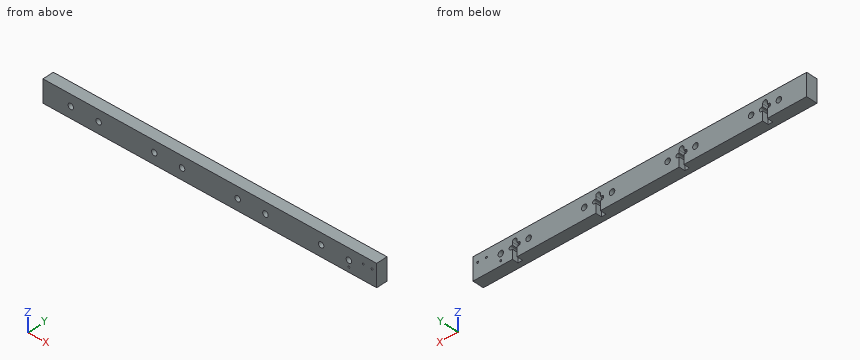
from build123d import *

# Parameters (mm, degrees)
SKETCH1_W                = 360
SKETCH1_H                = 24
BOSS_EXTRUDE1_DEPTH      = 12
CUT_EXTRUDE1_REACH       = 182.798
SKETCH2_R                = 3
CUT_EXTRUDE2_DEPTH       = 8
CUT_EXTRUDE3_DEPTH       = 6.5
LPATTERN1_COUNT          = 4
LPATTERN1_PITCH          = 90
F_2_0_2_DIAMETER_HOLE1_D = 2


with BuildPart() as part:
    # Sketch1 → Boss-Extrude1 (new body)
    with BuildSketch(Plane(origin=(0, 0, 0), x_dir=(1, 0, 0), z_dir=(0, 1, 0))):
        Rectangle(SKETCH1_W, SKETCH1_H)
    extrude(amount=BOSS_EXTRUDE1_DEPTH)

    # Sketch2 → Cut-Extrude1 (cut, up to next)
    with BuildSketch(Plane(origin=(0, 12, 0), x_dir=(1, 0, 0), z_dir=(0, 1, 0)), mode=Mode.PRIVATE) as cut_extrude1_sk1:
        with Locations(Location((-150, 0, 0), (0, 0, 270))):
            Circle(SKETCH2_R)
    cut_extrude1_tool1 = extrude(cut_extrude1_sk1.sketch, amount=-CUT_EXTRUDE1_REACH, mode=Mode.PRIVATE) & part.part
    # Sketch2 → Cut-Extrude1 (cut, up to next)
    with BuildSketch(Plane(origin=(0, 12, 0), x_dir=(1, 0, 0), z_dir=(0, 1, 0)), mode=Mode.PRIVATE) as cut_extrude1_sk2:
        with Locations(Location((-120, 0, 0), (0, 0, 270))):
            Circle(SKETCH2_R)
    cut_extrude1_tool2 = extrude(cut_extrude1_sk2.sketch, amount=-CUT_EXTRUDE1_REACH, mode=Mode.PRIVATE) & part.part
    cut_extrude1_1 = cut_extrude1_tool1.solids().sort_by_distance((-150, 12, 0))[0]
    add(cut_extrude1_1, mode=Mode.SUBTRACT)
    cut_extrude1_2 = cut_extrude1_tool2.solids().sort_by_distance((-120, 12, 0))[0]
    add(cut_extrude1_2, mode=Mode.SUBTRACT)
    cut_extrude1 = cut_extrude1_1 + cut_extrude1_2  # Cut-Extrude1 as one shape, for the pattern or mirror that repeats it

    # Sketch11 → Cut-Extrude2 (cut)
    with BuildSketch(Plane(origin=(-63.484819349, 12, 93.481372316), x_dir=(-1, 0, 0), z_dir=(0, 1, 0))):
        with BuildLine():
            Line((67.515180651, -91.481372316), (75.515180651, -91.481372316))
            ThreePointArc((75.515180651, -91.481372316), (77.515180651, -93.481372316), (75.515180651, -95.481372316))
            Line((75.515180651, -95.481372316), (67.515180651, -95.481372316))
            ThreePointArc((67.515180651, -95.481372316), (65.515180651, -93.481372316), (67.515180651, -91.481372316))
        make_face()
    cut_extrude2 = extrude(amount=-CUT_EXTRUDE2_DEPTH, mode=Mode.SUBTRACT)

    # Sketch13 → Cut-Extrude3 (cut)
    with BuildSketch(Plane(origin=(-63.484819349, 12, 93.481372316), x_dir=(-1, 0, 0), z_dir=(0, 1, 0))):
        with BuildLine():
            Line((74.015180651, -88.481372316), (74.015180651, -142.11123171))
            ThreePointArc((74.015180651, -142.11123171), (71.515180651, -144.61123171), (69.015180651, -142.11123171))
            Line((69.015180651, -142.11123171), (69.015180651, -88.481372316))
            ThreePointArc((69.015180651, -88.481372316), (71.515180651, -85.981372316), (74.015180651, -88.481372316))
        make_face()
    cut_extrude3 = extrude(amount=-CUT_EXTRUDE3_DEPTH, mode=Mode.SUBTRACT)

    # LPattern1: Cut-Extrude1, Cut-Extrude2, Cut-Extrude3 ×4
    with Locations(*[(i * LPATTERN1_PITCH, 0, 0) for i in range(1, LPATTERN1_COUNT)]):
        add(cut_extrude1, mode=Mode.SUBTRACT)
        add(cut_extrude2, mode=Mode.SUBTRACT)
        add(cut_extrude3, mode=Mode.SUBTRACT)

    # Ø2.0 (2) Diameter Hole1 (through all)
    with Locations(Plane.XZ):
        with Locations((165.5, 4), (175, 4), (150, -7)):
            Hole(F_2_0_2_DIAMETER_HOLE1_D / 2)


solid = part.part
Check sheet for the modelled part. Datum: model origin and axes. Units: mm. Round coordinates to 2 decimals unless told otherwise and drop trailing zeros. Order: outer loops, then holes, each group sorted by start corner. A loop starts at its lowest first (then second) coordinate and runs counter-clockwise, first axis right, second up.
(1) Cross-section at A-A, the plane x = 120. Enter the section's corners in (y, z).
(2) Cross-section at B-B, the plane y = 7.5. State how many separate pieces and enclosed holes the cut face has, and give its area (3 significant figures).
(3) Scan lines: probe 1 along Z at (x, y) = (30, 5.5); probe 2 along X at (y, z) = (10.5, -5.5); probe 3 along Z at (x, y) = (175, 9). Record each from-to range of solid material in increasing order.
(4) Go/stop test with flat-tipped pins: P1, Ø1.5, axis at x = 136, z = 4.5, coming from the +Y side; P2, Ø3.5, axis at x = 60, z = 0, coming from the -Y side. Record where each tip stops, or that it passes through.
Check sheet entries:
1. outline: (0, -12) - (12, -12) - (12, -3) - (0, -3) - close; (0, 3) - (12, 3) - (12, 12) - (0, 12) - close
2. separate pieces: 1
2. enclosed holes: 11
2. area: 7,930 mm2
3. probe 1: z = -12 to -3, 3 to 12
3. probe 2: x = -180 to -137.5, -132.5 to -47.5, -42.5 to 42.5, 47.5 to 132.5, 137.5 to 180
3. probe 3: z = -12 to 3, 5 to 12
4. P1: stops at y = 5.5
4. P2: passes through
